Read the model definition and answer for the solid it produces. Units are mm, in the model's axes. A direction names the side the tool comes from. Coordinates: 2 decimals unless noted, no trailing zeros. Write each loop counter-clockwise with the first axis right and the second up, starting at its lowest first coordinate (ties: lowest second). Pieces come first, ordered by that corner, then holes.
(1) Given pin 1 (1.7 mm diameter, centred on x = 78.5, z = 4, fed in from -Y) (3 decimals); pin 2 (1.8 mm diameter, centred on x = 101.6, y = 0, fed in from -Z); pin 3 (2 mm diameter, centred on y = 8.5, z = 2, fed in from -X); pin 4 (0.9 mm diameter, centred on y = -10.5, z = 4, fed in from +X) (3 decimals), each flat-ended and moving along its own axis, determine where each tip first touches the part or whether it passes through.
(2) Determine the mould class of faces 5 (the cylindrical face through (111.123, 0.209, 2.843)), 6 (the flat face through (1, -9.525, 3)), 7 (the flat face through (-1, 9.525, 3)), 8 (the flat face through (55, -12.484, 3)) for opening direction X: pulls with the +X half, pulls with the -X half, needs draft (parallel to the pull), parting line crosses it, or undercut.
(3) The part is cut by section C-C, the plane y = -7.5. Determine the outline of the cut face in (x, z).
(4) Which of the six approach directions +Z, -Z, +X, -X, +Y, -Y give full straight-line access (tool end or side, diameter ignored) to faces 1 (the flat face through (81, 9.525, 3)), 2 (the flat face through (81, -9.525, 3)), 3 (the flat face through (-81, -9.525, 3)), 4 (the flat face through (-81, 9.525, 3))?
(5) The part is cut by section A-A, the plane z = 2.6. Determine the outline of the cut face in (x, y) (3 decimals), and give its area (3 significant figures).
(6) Straight lines are drawn through the part: line 1 along X through (y, z) = (10.75, 2.35) (3 decimals); line 2 along Y through (x, z) = (-25.4, 3.75) (3 decimals); line 3 along X through (y, z) = (0.5, 4.45). For each, find the intervals that lie inside material, in ascending order.
(7) The part is cut by section B-B, the plane x = -16.5. Determine the outline of the cut face in (y, z) (3 decimals), and give its area (3 significant figures).
```python
from build123d import *

# Parameters (mm, degrees)
SKETCH1_R             = 1.4732
BOSS_EXTRUDE1_DEPTH   = 5.7658
F_4_CLEARANCE_HOLE1_D = 2.9464
SKETCH5_W             = 9.525
SKETCH5_H             = 2.9591
BOSS_EXTRUDE2_DEPTH   = 5.7658


with BuildPart() as part:
    # Sketch1 → Boss-Extrude1 (new body)
    with BuildSketch(Plane.XY):
        with BuildLine():
            Line((-101.6, 9.525), (101.6, 9.525))
            ThreePointArc((101.6, 9.525), (111.125, 0), (101.6, -9.525))
            Line((101.6, -9.525), (-101.6, -9.525))
            ThreePointArc((-101.6, -9.525), (-111.125, 0), (-101.6, 9.525))
        make_face()
        with Locations((-101.6, 0)):
            Circle(SKETCH1_R, mode=Mode.SUBTRACT)
        with Locations((101.6, 0)):
            Circle(SKETCH1_R, mode=Mode.SUBTRACT)
    extrude(amount=BOSS_EXTRUDE1_DEPTH)

    # #4 Clearance Hole1 (through all)
    with Locations(Plane.XY.offset(5.7658)):
        with Locations((-25.4, 0), (12.7, 0), (0, 0)):
            Hole(F_4_CLEARANCE_HOLE1_D / 2)

    # Sketch5 → Boss-Extrude2 (add)
    with BuildSketch(Plane.XY.offset(5.7658)):
        with Locations((55.5625, 11.00455)):
            Rectangle(SKETCH5_W, SKETCH5_H)
        with Locations((-55.5625, 11.00455)):
            Rectangle(SKETCH5_W, SKETCH5_H)
        with Locations((-55.5625, -11.00455)):
            Rectangle(SKETCH5_W, SKETCH5_H)
        with Locations((55.5625, -11.00455)):
            Rectangle(SKETCH5_W, SKETCH5_H)
    extrude(amount=-BOSS_EXTRUDE2_DEPTH)


solid = part.part
```
Computed:
1. pin 1: stops at y = -9.525
1. pin 2: passes through
1. pin 3: stops at x = -107.47
1. pin 4: stops at x = 60.325
2. face 5: pulls with the +X half
2. face 6: undercut
2. face 7: undercut
2. face 8: needs draft
3. outline: (-107.47, 0) - (107.47, 0) - (107.47, 5.77) - (-107.47, 5.77) - close
4. face 1: +Z, -Z, +X, +Y
4. face 2: +Z, -Z, +X, -Y
4. face 3: +Z, -Z, -X, -Y
4. face 4: +Z, -Z, -X, +Y
5. outline: (-101.6, -9.525) - (-60.325, -9.525) - (-60.325, -12.484) - (-50.8, -12.484) - (-50.8, -9.525) - (50.8, -9.525) - (50.8, -12.484) - (60.325, -12.484) - (60.325, -9.525) - (101.6, -9.525) arc R9.525 ccw to (101.6, 9.525) - (60.325, 9.525) - (60.325, 12.484) - (50.8, 12.484) - (50.8, 9.525) - (-50.8, 9.525) - (-50.8, 12.484) - (-60.325, 12.484) - (-60.325, 9.525) - (-101.6, 9.525) arc R9.525 ccw to start; hole circle Ø2.946 at (-101.6, 0); hole circle Ø2.946 at (-25.4, 0); hole circle Ø2.946 at (0, 0); hole circle Ø2.946 at (12.7, 0); hole circle Ø2.946 at (101.6, 0)
5. area: 4,230 mm2
6. line 1: x = -60.325 to -50.8, 50.8 to 60.325
6. line 2: y = -9.525 to -1.473, 1.473 to 9.525
6. line 3: x = -111.11 to -102.99, -100.21 to -26.79, -24.01 to -1.39, 1.39 to 11.31, 14.09 to 100.21, 102.99 to 111.11
7. outline: (-9.525, 0) - (9.525, 0) - (9.525, 5.766) - (-9.525, 5.766) - close
7. area: 110 mm2
